Answer from the drawing. Dimensions are ordinates in mm from the lowest x, y and z of the part. Round coordinates to 2 decimals unless told otherwise and drop trailing zeros. Loops run counter-clockwise (first coordinate to the right, second up) from the corner with the lowest first, then second, coordinate; pieces in that order, holes last.
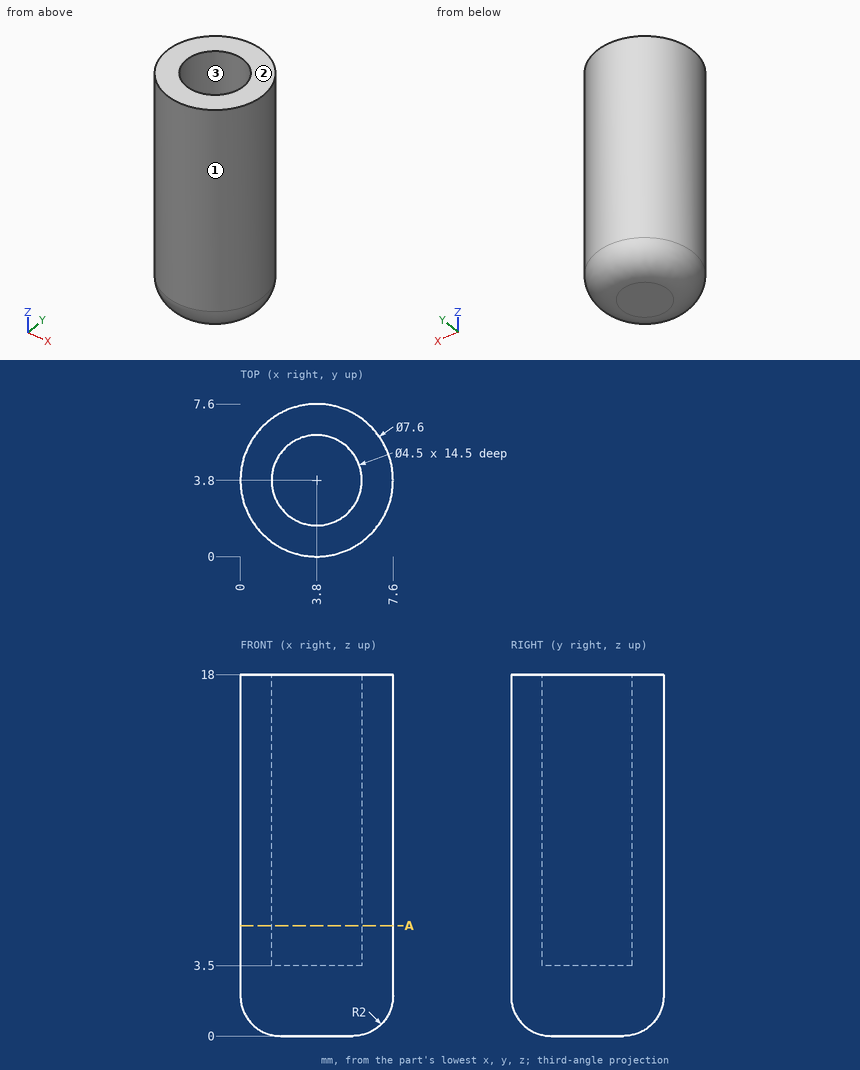
1. Given pin 1 (1.5 mm diameter, centred on y = 5, z = 11.5, fed in from +X); pin 2 (1 mm diameter, centred on x = 1, z = 12.5, fed in from -Y); pin 3 (2 mm diameter, centred on x = 4.5, y = 4.5, fed in from +Z), each flat-ended and moving along its own axis, determine where each tip first touches the part or whether it passes through.
Answer key:
pin 1: stops at x = 7.57
pin 2: stops at y = 0.78
pin 3: stops at z = 3.5
2. Determine the mould class of the marked faces 1, 2 and 3 for opening direction X: +X half, -X half, draft (parallel to the pull), parting line (faces both ways), or undercut.
Answer key:
face 1: parting line
face 2: draft
face 3: undercut
3. Find section A-A (z = 5.5). Write down the section's boundary in (x, y).
Answer key:
outline: circle Ø7.6 at (3.8, 3.8); hole circle Ø4.5 at (3.8, 3.8)
4. Consider probe 1 along X at (y, z) = (3.75, 8.75); probe 2 along X at (y, z) = (3, 9). Determine where each line is inside the solid, lowest interval first.
Answer key:
probe 1: x = 0 to 1.55, 6.05 to 7.6
probe 2: x = 0.09 to 1.7, 5.9 to 7.51
